Print and shaded views of the part. All mm, measured from the part's lowest x, y and z. Give positions to 0.01 mm unless a question says otherwise; leave off trailing zeros. Write each loop counter-clockwise with the first axis right and the second up, starting at its lowest first coordinate (ties: lowest second). Pieces come first, ordered by that corner, then holes. Notation, with made-up numbers: (74.25, 6.25) -> (78.25, 6.25) arc R28 cw to (78.25, 28.25) -> close; hole circle Ø1 at (-18, 74.25). An arc over 180 degrees is marked (long way). Put each result on its own line as item: value.
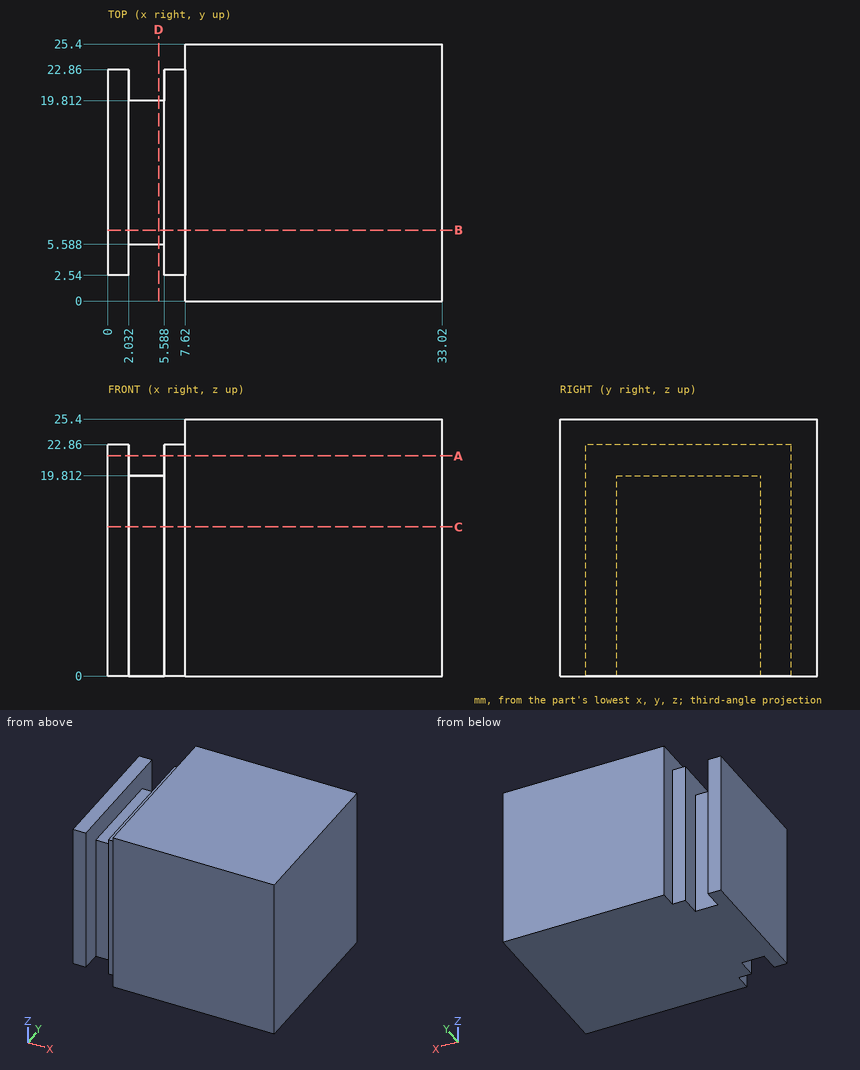
1) Pin check, flat tips, straight feed: pin 1 (1 mm diameter, centred on x = 1, z = 7, fed in from +Y); pin 2 (1.6 mm diameter, centred on x = 1, z = 15, fed in from -Y); pin 3 (1.6 mm diameter, centred on x = 0.5, y = 8.5, fed in from +Z). Stop position of each tip, or through.
Filled sheet:
pin 1: y = 22.86
pin 2: y = 2.54
pin 3: z = 22.86
2) Slice it at C-C (z = 14.75). Write the cut outline in (x, y).
Filled sheet:
outline: (0, 2.54) -> (2.03, 2.54) -> (2.03, 5.59) -> (5.59, 5.59) -> (5.59, 2.54) -> (7.62, 2.54) -> (7.62, 0) -> (33.02, 0) -> (33.02, 25.4) -> (7.62, 25.4) -> (7.62, 22.86) -> (5.59, 22.86) -> (5.59, 19.81) -> (2.03, 19.81) -> (2.03, 22.86) -> (0, 22.86) -> close
3) Wall check: L1, parallel to X at y = 21, z = 6.75; L2, parallel to Z at x = 4, y = 16; L3, parallel to Z at x = 7, y = 17.5. Give the ranges that are in metal, low to high.
Filled sheet:
L1: 0 to 2.03, 5.59 to 33.02
L2: 0 to 19.81
L3: 0 to 22.86
4) Slice it at A-A (z = 21.75). Write the cut outline in (x, y), plus the area to 3 significant figures.
Filled sheet:
outline: (0, 2.54) -> (2.03, 2.54) -> (2.03, 22.86) -> (0, 22.86) -> close; (5.59, 2.54) -> (7.62, 2.54) -> (7.62, 0) -> (33.02, 0) -> (33.02, 25.4) -> (7.62, 25.4) -> (7.62, 22.86) -> (5.59, 22.86) -> close
area: 728 mm2
5) Slice it at B-B (y = 7). Write the cut outline in (x, z).
Filled sheet:
outline: (0, 0) -> (33.02, 0) -> (33.02, 25.4) -> (7.62, 25.4) -> (7.62, 22.86) -> (5.59, 22.86) -> (5.59, 19.81) -> (2.03, 19.81) -> (2.03, 22.86) -> (0, 22.86) -> close
6) Slice it at D-D (x = 5). Write the cut outline in (y, z).
Filled sheet:
outline: (5.59, 0) -> (19.81, 0) -> (19.81, 19.81) -> (5.59, 19.81) -> close
